```python
from build123d import *

# Parameters (mm, degrees)
SKETCH1_R           = 2
BOSS_EXTRUDE1_DEPTH = 20
SKETCH2_W           = 31.562668847
SKETCH2_H           = 7.62
CUT_EXTRUDE1_DEPTH  = 15.24
SKETCH5_R           = 2.11
CUT_EXTRUDE2_DEPTH  = 10.414


with BuildPart() as part:
    # Sketch1 → Boss-Extrude1 (new body)
    with BuildSketch(Plane.XY):
        Polygon((-16.147505616, -28.306513497), (-16.147505616, -35.926513497), (-47.710174463, -35.926513497), (-47.710174463, -28.306513497), (-47.710174463, -24.496513497), (-16.147505616, -24.496513497), align=None)
        with Locations((-40.868568225, -32.116513497)):
            Circle(SKETCH1_R, mode=Mode.SUBTRACT)
        with Locations((-23.868568225, -32.116530453)):
            Circle(SKETCH1_R, mode=Mode.SUBTRACT)
    extrude(amount=BOSS_EXTRUDE1_DEPTH)

    # Sketch2 → Cut-Extrude1 (cut)
    with BuildSketch(Plane.XY.offset(20)):
        with Locations((-31.92884004, -32.116513497)):
            Rectangle(SKETCH2_W, SKETCH2_H)
    extrude(amount=-CUT_EXTRUDE1_DEPTH, mode=Mode.SUBTRACT)

    # Sketch5 → Cut-Extrude2 (cut)
    with BuildSketch(Plane(origin=(0, -24.496513497, 0), x_dir=(1, 0, 0), z_dir=(0, 1, 0))):
        with Locations(Location((-23.868568225, -16.19, 0), (0, 0, 270))):
            Circle(SKETCH5_R)
        with Locations(Location((-40.868568225, -16.19, 0), (0, 0, 270))):
            Circle(SKETCH5_R)
    extrude(amount=-CUT_EXTRUDE2_DEPTH, mode=Mode.SUBTRACT)


solid = part.part
```
CAD build for the part. Positions are in the model's coordinates, mm. A direction names the side the tool comes from. Coordinates: 2 decimals unless noted, no trailing zeros. Order: outer loops, then holes, each group sorted by start corner. A loop starts at its lowest first (then second) coordinate and runs counter-clockwise, first axis right, second up. Notation, with made-up numbers: M 18.25,-16.5 L 45.25,-16.5 A21 cw 45.25,-7.5 Z; hole C 75.25,84.25 d9. An arc over 180 degrees is marked long. Answer as CSV lines item,"result".
1) Cut at A-A (z = 16.19). List the corners of the cut face in (x, y), then the cut area to 3 significant figures.
Verdict:
outline,"M -47.71,-28.31 L -42.98,-28.31 L -42.98,-24.5 L -47.71,-24.5 Z; M -38.76,-28.31 L -25.98,-28.31 L -25.98,-24.5 L -38.76,-24.5 Z; M -21.76,-28.31 L -16.15,-28.31 L -16.15,-24.5 L -21.76,-24.5 Z"
area,"88.1 mm2"
2) 3-axis set-ups, long thin cutter, end or side, ignore diameter. For faces 4 (the flat face through (-32, -32, 4.76)), 5 (the cylindrical face through (-24.3, -34.07, 2.35)): which of +Z, -Z, +X, -X, +Y, -Y reach the whole face in a straight line?
Verdict:
face 4,"+Z, +X, -X, -Y"
face 5,"+Z, -Z"
3) Cut at B-B (y = -33.5). List the corners of the cut face in (x, z).
Verdict:
outline,"M -47.71,0 L -42.31,0 L -42.31,4.76 L -47.71,4.76 Z; M -39.42,0 L -25.31,0 L -25.31,4.76 L -39.42,4.76 Z; M -22.42,0 L -16.15,0 L -16.15,4.76 L -22.42,4.76 Z"
4) Cut at C-C (x = -22.5). List the corners of the cut face in (y, z), then the cut area to 3 significant figures.
Verdict:
outline,"M -35.93,0 L -33.57,0 L -33.57,4.76 L -35.93,4.76 Z; M -30.66,0 L -24.5,0 L -24.5,14.58 L -28.31,14.58 L -28.31,4.76 L -30.66,4.76 Z; M -28.31,17.8 L -24.5,17.8 L -24.5,20 L -28.31,20 Z"
area,"86.3 mm2"
5) Mould opens along X. For faces 1 (the cylindrical face through (-38.96, -31.52, 2.35)), 2 (the flat face through (-47.71, -28, 8)), 3 (the flat face through (-32, -28.307, 12)) say: released by +X, released by -X, zero draft, split by the parting line, or undercut.
Verdict:
face 1,"undercut"
face 2,"released by -X"
face 3,"zero draft"
6) Drill centre lines: L1, parallel to X at y = -26.9, z = 16.19; L2, parallel to X at y = -32, z = 1; L3, parallel to Z at x = -40, y = -29.5. Where is each one in solid material? Low to high. Write a range as from..to.
Verdict:
L1,"-47.71..-42.98, -38.76..-25.98, -21.76..-16.15"
L2,"-47.71..-42.87, -38.87..-25.87, -21.87..-16.15"
L3,"0..4.76"
7) Flat gauge pins, fed straight in: P1, Ø3, axis at x = -31.5, y = -31.5, coming from the -Z side; P2, Ø3, axis at x = -40.87, y = -32.12, coming from the -Z side; P3, Ø12, axis at x = -37.5, z = 14.5, coming from the -Y side; P4, Ø6, axis at x = -25, y = -33, coming from the +Z side. Where does each tip first touch, or does it go through?
Verdict:
P1,"z = 0"
P2,"through"
P3,"y = -28.31"
P4,"z = 4.76"
8) Cut at D-D (y = -26). List the corners of the cut face in (x, z), then the cut area to 3 significant figures.
Verdict:
outline,"M -47.71,0 L -16.15,0 L -16.15,20 L -47.71,20 Z; hole C -40.87,16.19 d4.22; hole C -23.87,16.19 d4.22"
area,"603 mm2"
